Check sheet for the drawn part. Datum: minimum x, y, z corner. Units: mm. Give positions to 0.01 mm unless a question says otherwise; leave off trailing zeros. Loops run counter-clockwise (first coordinate to the right, second up) from the corner with the lowest first, then second, coordinate; pieces in that order, holes last. Notation, with made-up numbers: (-8, 83.5) - (33, 83.5) arc R26 cw to (33, 103.5) - close; hole circle Ø5 at (-14.75, 7). An arc over 180 degrees is marked (long way). Use a Markdown table: item, result. Add a question column.
1. Cross-section at C-C on x = 63. Enter the section's corners in (y, z).
2. Draft check along X on the marked faces 1 and 2. Enter one of: pulls with the +X half, pulls with the -X half, needs draft (parallel to the pull), parting line crosses it, or undercut.
3. Cross-section at D-D on y = 2. Enter the section's corners in (x, z).
4. Material ranges on L1, parallel to Y at x = 34.5, z = 4.25; L2, parallel to X at y = 20.25, z = 1; L3, parallel to X at y = 13, z = 7.75, recorded low to high.
5. Depth check by flat-ended pin: P1, Ø2, axis at x = 71, z = 8, coming from the +Y side. Enter the tip coordinate at first touch or a pass-through.
6. Cross-section at B-B on y = 20.5. Enter the section's corners in (x, z).
7. Cross-section at A-A on z = 8. Enter the section's corners in (x, y).
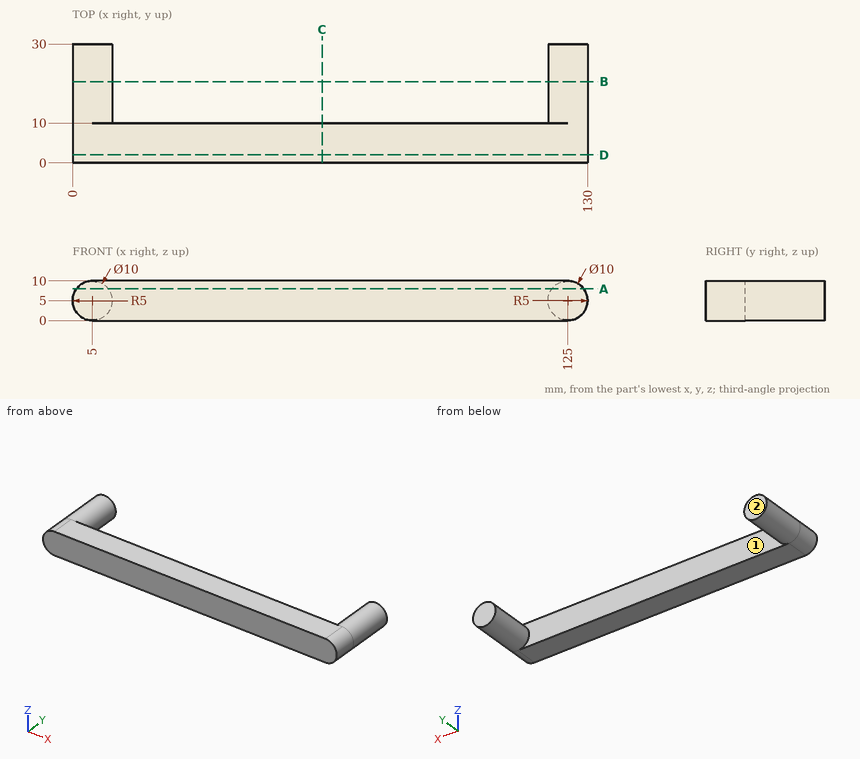
Values found:
| question | item | result |
|---|---|---|
| 1 | outline | (0, 0) - (10, 0) - (10, 10) - (0, 10) - close |
| 2 | face 1 | undercut |
| 2 | face 2 | needs draft |
| 3 | outline | (5, 0) - (125, 0) arc R5 ccw to (125, 10) - (5, 10) arc R5 ccw to start |
| 4 | L1 | y = 0 to 10 |
| 4 | L2 | x = 2 to 8, 122 to 128 |
| 4 | L3 | x = 0.82 to 9.18, 120.82 to 129.18 |
| 5 | P1 | stops at y = 10 |
| 6 | outline | circle Ø10 at (5, 5); circle Ø10 at (125, 5) |
| 7 | outline | (1, 0) - (129, 0) - (129, 30) - (121, 30) - (121, 10) - (9, 10) - (9, 30) - (1, 30) - close |
